```python
from build123d import *

# Parameters (mm, degrees)
F0_W     = 38
F0_H     = 5
F1_DEPTH = 15
F2_R     = 1.5
F3_DEPTH = 8
F4_W     = 38
F4_H     = 7.5
F5_DEPTH = 10
F6_R     = 2.5
F7_DEPTH = 10


with BuildPart() as f1:
    # F0 (on Front) → F1 (new body)
    with BuildSketch(Plane.XZ):
        Rectangle(F0_W, F0_H)
    extrude(amount=F1_DEPTH)

    # F2 (on face) → F3 (cut)
    with BuildSketch(Plane.XZ):
        with Locations((-10.5, 0)):
            Circle(F2_R)
        with Locations((10.5, 0)):
            Circle(F2_R)
    extrude(amount=F3_DEPTH, mode=Mode.SUBTRACT)

    # F4 (on face) → F5 (join)
    with BuildSketch(Plane.XY.offset(2.5)):
        with Locations((0, -11.25)):
            Rectangle(F4_W, F4_H)
    extrude(amount=F5_DEPTH)

    # F6 (on face) → F7 (cut)
    with BuildSketch(Plane.XZ.offset(15)):
        with Locations((-14, 6.5)):
            Circle(F6_R)
        with Locations((14, 6.5)):
            Circle(F6_R)
    extrude(amount=-F7_DEPTH, mode=Mode.SUBTRACT)


solid = f1.part
```
Build history of the part. All positions in model axes, mm. A direction names the side the tool comes from. Round coordinates to 2 decimals unless told otherwise and drop trailing zeros. Write each loop counter-clockwise with the first axis right and the second up, starting at its lowest first coordinate (ties: lowest second). Pieces come first, ordered by that corner, then holes. Notation, with made-up numbers: (53.5, 24) - (101.5, 24) arc R23 cw to (101.5, 51) - close; hole circle Ø4 at (80.5, -6.75). An arc over 180 degrees is marked (long way). Answer as CSV lines item,"result".
Q1. Cut at A-A (x = -14). Write the cut outline in (y, z).
Report:
outline,"(-15, -2.5) - (0, -2.5) - (0, 2.5) - (-7.5, 2.5) - (-7.5, 4) - (-15, 4) - close; (-15, 9) - (-7.5, 9) - (-7.5, 12.5) - (-15, 12.5) - close"
Q2. Drop flat-ended pins along their axis: pin 1 (2 mm diameter, centred on x = -2.5, z = 8.5, fed in from +Y); pin 2 (1.5 mm diameter, centred on x = -10.5, z = 0, fed in from +Y). Give the stop position or say it passes through.
Report:
pin 1,"stops at y = -7.5"
pin 2,"stops at y = -8"
Q3. Cut at C-C (y = -1.5). Write the cut outline in (x, z).
Report:
outline,"(-19, -2.5) - (19, -2.5) - (19, 2.5) - (-19, 2.5) - close; hole circle Ø3 at (-10.5, 0); hole circle Ø3 at (10.5, 0)"
Q4. Drill centre lines: probe 1 along Z at (x, y) = (-14, -12); probe 2 along X at (y, z) = (-3.5, 1.25); probe 3 along X at (y, z) = (-2.75, -0.75). Where is each one in solid material? Low to high. Write a range as [from, to].
Report:
probe 1,"z = [-2.5, 4], [9, 12.5]"
probe 2,"x = [-19, -11.33], [-9.67, 9.67], [11.33, 19]"
probe 3,"x = [-19, -11.8], [-9.2, 9.2], [11.8, 19]"
Q5. Pull direction Z, two halves, no side cores. Call faces 4 (the flat face through (0, -7, -2.5)), 5 (the flat face through (0, 0, 0)), 6 (the cylindrical face through (-12, -4, 0)): +Z half, -Z half, draft (parallel to the pull), parting line (faces both ways), or undercut.
Report:
face 4,"-Z half"
face 5,"draft"
face 6,"undercut"
Q6. Tool access for faces 1 (the flat face through (0, -15, 5)), 2 (the flat face through (-11, -8, 0)), 3 (the flat face through (0, -7.5, 7)): list every direction of +Z, -Z, +X, -X, +Y, -Y with a clear straight run to the whole face (end or side of a thin tool).
Report:
face 1,"+Z, -Z, +X, -X, -Y"
face 2,"+Y"
face 3,"+Z, +X, -X, +Y"
Q7. Cut at D-D (z = 0). Write the cut outline in (x, y).
Report:
outline,"(-19, -15) - (19, -15) - (19, 0) - (12, 0) - (12, -8) - (9, -8) - (9, 0) - (-9, 0) - (-9, -8) - (-12, -8) - (-12, 0) - (-19, 0) - close"
Q8. Cut at B-B (z = 6.5). Write the cut outline in (x, y).
Report:
outline,"(-19, -15) - (-16.5, -15) - (-16.5, -7.5) - (-19, -7.5) - close; (-11.5, -15) - (11.5, -15) - (11.5, -7.5) - (-11.5, -7.5) - close; (16.5, -15) - (19, -15) - (19, -7.5) - (16.5, -7.5) - close"
